Geometry: final body of the model. Coordinates: model frame, mm. A direction names the side the tool comes from. Give positions to 0.01 mm unless a question says otherwise; leave off trailing zeros. Write each loop counter-clockwise with the first axis right and the second up, starting at its lowest first coordinate (ties: lowest second). Pieces come first, ordered by that corner, then holes. Notation, with made-up numbers: M 46.25,77.25 L 101.25,77.25 A23 ccw 101.25,100.25 Z; hole C 48,-25.75 d6. An arc over 180 degrees is marked long. Answer as a JSON object with one key per item and string values.
from build123d import *

# Parameters (mm, degrees)
F0_W      = 88
F0_H      = 27.705
F2_SIZE   = 1
F3_R      = 12.45
F4_DEPTH  = 2
F5_R      = 12.465
F6_DEPTH  = 2
F7_R      = 2
F8_DEPTH  = 10
F9_R      = 6
F10_DEPTH = 5
F11_R     = 2.98
F12_DEPTH = 23.35
F13_R     = 2
F14_DEPTH = 5


with BuildPart() as f1:
    # F0 (on Front) → F1 (revolve)
    with BuildSketch(Plane.XZ):
        with Locations((-2.593532, 13.8525)):
            Rectangle(F0_W, F0_H)
    revolve(axis=Axis((-2.593532, 0, 0), (-1, 0, 0)))

    # F2
    f2_edges = [f1.edges().sort_by_distance(p)[0] for p in [
        (-46.593532, 0, -27.705),
        (41.406468, 0, -27.705),
    ]]
    chamfer(f2_edges, length=F2_SIZE)

    # F3 (on face) → F4 (join)
    with BuildSketch(Plane.YZ.offset(41.406468)):
        Circle(F3_R)
    extrude(amount=F4_DEPTH)

    # F5 (on face) → F6 (join)
    with BuildSketch(Plane(origin=(-46.593532, 0, 0), x_dir=(0, -1, 0), z_dir=(-1, 0, 0))):
        Circle(F5_R)
    extrude(amount=F6_DEPTH)

    # F7 (on face) → F8 (cut)
    with BuildSketch(Plane(origin=(-46.593532, 0, 0), x_dir=(0, -1, 0), z_dir=(-1, 0, 0))):
        with Locations((0, 20)):
            Circle(F7_R)
        with Locations((-20, 0)):
            Circle(F7_R)
        with Locations((0, -20)):
            Circle(F7_R)
        with Locations((20, 0)):
            Circle(F7_R)
    extrude(amount=-F8_DEPTH, mode=Mode.SUBTRACT)

    # F9 (on face) → F10 (cut)
    with BuildSketch(Plane.YZ.offset(43.406468)):
        Circle(F9_R)
    extrude(amount=-F10_DEPTH, mode=Mode.SUBTRACT)

    # F11 (on face) → F12 (join)
    with BuildSketch(Plane.YZ.offset(38.406468)):
        Circle(F11_R)
    extrude(amount=F12_DEPTH)

    # F13 (on face) → F14 (cut)
    with BuildSketch(Plane.YZ.offset(41.406468)):
        with Locations((0, 20)):
            Circle(F13_R)
        with Locations((20, 0)):
            Circle(F13_R)
        with Locations((0, -20)):
            Circle(F13_R)
        with Locations((-20, 0)):
            Circle(F13_R)
    extrude(amount=-F14_DEPTH, mode=Mode.SUBTRACT)


solid = f1.part
1) Line query: line 1 (Y direction, x = -40.5, z = -0.5); line 2 (X direction, y = 4, z = 19.5); line 3 (Z direction, x = -7.5, y = -0.5). Output: solid intervals per line, ascending. Write a range as from..to.
Geometry check:
{"line 1": "y = -27.7..-21.94, -18.06..18.06, 21.94..27.7", "line 2": "x = -46.59..41.41", "line 3": "z = -27.7..27.7"}
2) Pull-direction query (Z, two-part tool) for faces 4 (the flat face through (-36.594, 0, 20)), 5 (the flat face through (61.756, 0, 0)), 6 (the cylindrical face through (42.39, -9.18, 8.41)); classes: pulls with the +Z half, pulls with the -Z half, needs draft (parallel to the pull), parting line crosses it, or undercut.
Geometry check:
{"face 4": "undercut", "face 5": "needs draft", "face 6": "parting line crosses it"}
3) Contact query for flat-ended pins moving along their axis: P1, Ø4.5, axis at y = -19, z = 0, coming from the +X side; P2, Ø3.5, axis at y = -2, z = -3, coming from the +X side; P3, Ø2, axis at x = -0.5, y = -2, coming from the +Z side; P4, Ø2.5, axis at y = 0, z = -20, coming from the -X side. Output: stop coordinate, or through.
Geometry check:
{"P1": "stops at x = 41.41", "P2": "stops at x = 61.76", "P3": "stops at z = 27.69", "P4": "stops at x = -36.59"}
4) Cut plane A-A on x = -10.5. Return loops of the section in (y, z) (3 decimals), and give its area (3 significant figures).
Geometry check:
{"outline": "C 0,0 d55.41", "area": "2,410 mm2"}
5) Set-up query: faces 1 (the cylindrical face through (-47.58, 2.7, -12.17)), 2 (the flat face through (-48.594, 0, 0)), 3 (the flat face through (36.406, 20, 0)). Return all of +Z, -Z, +X, -X, +Y, -Y with unobstructed straight access to the full face (end or side cutting, diameter ignored); none if empty.
Geometry check:
{"face 1": "-X", "face 2": "+Z, -Z, -X, +Y, -Y", "face 3": "+X"}
